Autodesk Inventor part; units mm, degrees
ref_plane "YZ Plane" through (0, 0, 0) normal (1, 0, 0) x (0, 1, 0)
ref_plane "XZ Plane" through (0, 0, 0) normal (0, 1, 0) x (-1, 0, 0)
ref_plane "XY Plane" through (0, 0, 0) normal (0, 0, 1) x (1, 0, 0)
sketch "Sketch1" plane through (0, 0, 0) normal (0, 0, 1) x (1, 0, 0)
  line L0 (-25.4, 25.4) -> (25.4, 25.4)
  line L1 (25.4, 25.4) -> (25.4, -25.4)
  line L2 (25.4, -25.4) -> (-25.4, -25.4)
  line L3 (-25.4, -25.4) -> (-25.4, 25.4)
  line L4 (24.638, 24.638) -> (-24.638, 24.638)
  line L5 (-24.638, 24.638) -> (-24.638, -24.638)
  line L6 (-24.638, -24.638) -> (24.638, -24.638)
  line L7 (24.638, -24.638) -> (24.638, 24.638)
  point P0 (0, 0)
  point P1 (0, 25.4)
  point P2 (25.4, 0)
  dimension "d0" = 50.8
  dimension "d1" = 50.8
  dimension "d2" = 0.762
extrude "Extrusion1" add sketch "Sketch1" along normal blind 279.4
sketch "Sketch2" plane through (25.4, -25.4, 0) normal (1, 0, 0) x (0, 0, -1)
  line L0 (0, 50.8) -> (-279.4, 50.8)
  line L1 (-279.4, 0) -> (-228.6, 0)
  line L2 (-228.6, 0) -> (-228.6, 50.8)
  line L3 (-228.6, 50.8) -> (-279.4, 50.8)
  line L4 (-279.4, 50.8) -> (-279.4, 0)
  line L5 (-278.638, 0.762) -> (-229.362, 0.762)
  line L6 (-229.362, 0.762) -> (-229.362, 50.038)
  line L7 (-229.362, 50.038) -> (-278.638, 50.038)
  line L8 (-278.638, 50.038) -> (-278.638, 0.762)
  point P0 (0, 25.4)
  dimension "d5" = 50.8
  dimension "d6" = 0.762
extrude "Extrusion2" add sketch "Sketch2" along normal blind 88.9
sketch "Sketch3" plane through (0, 0, 279.4) normal (0, 0, 1) x (1, 0, 0)
  point P0 (0, 0)
sketch "Sketch4" plane through (0, 0, 279.4) normal (0, 0, 1) x (1, 0, 0)
  line L0 (-25.4, -25.4) -> (114.3, -25.4)
  line L1 (114.3, 25.4) -> (63.5, 25.4)
  line L2 (63.5, 25.4) -> (63.5, -25.4)
  line L3 (63.5, -25.4) -> (114.3, -25.4)
  line L4 (114.3, -25.4) -> (114.3, 25.4)
  line L5 (113.538, 24.638) -> (64.262, 24.638)
  line L6 (64.262, 24.638) -> (64.262, -24.638)
  line L7 (64.262, -24.638) -> (113.538, -24.638)
  line L8 (113.538, -24.638) -> (113.538, 24.638)
  point P0 (0, 0)
  dimension "d9" = 50.8
  dimension "d10" = 0.762
extrude "Extrusion3" add sketch "Sketch4" along normal blind 177.8
properties part number "Side Rail"
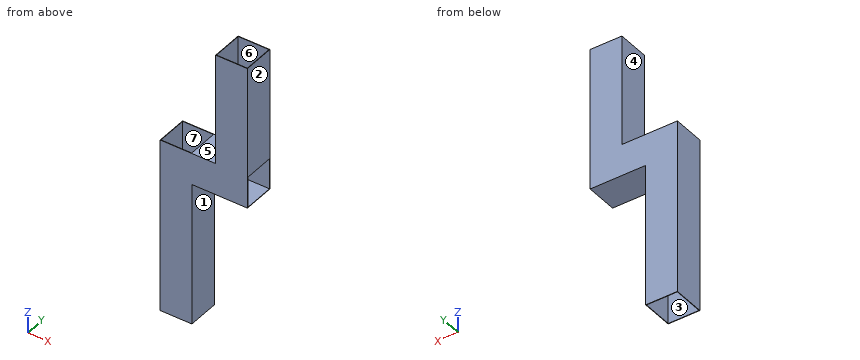
Input: part model. Units: mm. Frame: model coordinates. Face numbers are marked on the shaded views. A direction names the side the tool comes from. Round coordinates to 2 decimals unless told otherwise and drop trailing zeros. Order: outer loops, then holes, each group sorted by start corner. A loop starts at its lowest first (then second) coordinate and runs counter-clockwise, first axis right, second up. Notation, with made-up numbers: (54.25, -4) - (70.25, -4) arc R18 ccw to (70.25, 13) - close; hole circle Ø3 at (-15.75, 9). An arc over 180 degrees is marked (long way). One line per question, with ' | ' between items. Start each with the question number.
1) Ray query, probe 1 along Y at (x, z) = (95, 422.5); probe 2 along Z at (x, y) = (47, -5). Return the intervals inside material, ascending.
2) Cut plane D-D, the plane x = 9. Return the cut outline in (y, z), then the cut area to 3 significant figures.
3) Pull-direction query (X, two-part tool) for the marked faces 4, 5, 6 and 7; classes: +X half, -X half, draft (parallel to the pull), parting line (faces both ways), or undercut.
4) Set-up query: the marked faces 1, 2 and 3. Return all of +Z, -Z, +X, -X, +Y, -Y with unobstructed straight access to the full face (end or side cutting, diameter ignored); none if empty.
5) Cut plane C-C, the plane z = 425.5. Return the cut outline in (x, y), then the cut area to 3 significant figures.
6) Cut plane B-B, the plane x = 71. Return the cut outline in (y, z).
7) Contact query for flat-ended pins moving along their axis: P1, Ø15, axis at y = 6.5, z = 126, coming from the +X side; P2, Ø5, axis at x = 23.5, y = 11, coming from the +Z side; P3, Ø12, axis at x = 61, y = -7, coming from the -Z side. Output: stop coordinate, or through.
8) Cut plane A-A, the plane y = 16. Return the cut outline in (x, z), then the cut area to 3 significant figures.
Worked out:
1) probe 1: y = -25.4 to -24.64, 24.64 to 25.4 | probe 2: z = 228.6 to 229.36, 278.64 to 279.4
2) outline: (-25.4, 0) - (-24.64, 0) - (-24.64, 279.4) - (-25.4, 279.4) - close; (24.64, 0) - (25.4, 0) - (25.4, 279.4) - (24.64, 279.4) - close | area: 426 mm^2
3) face 4: -X half | face 5: draft | face 6: undercut | face 7: undercut
4) face 1: -Z, +X, +Y, -Y | face 2: +Z, -Z, +X, +Y, -Y | face 3: +Z, -Z
5) outline: (63.5, -25.4) - (114.3, -25.4) - (114.3, 25.4) - (63.5, 25.4) - close; hole (64.26, -24.64) - (113.54, -24.64) - (113.54, 24.64) - (64.26, 24.64) - close | area: 153 mm^2
6) outline: (-25.4, 228.6) - (25.4, 228.6) - (25.4, 457.2) - (24.64, 457.2) - (24.64, 279.4) - (-24.64, 279.4) - (-24.64, 457.2) - (-25.4, 457.2) - close; hole (-24.64, 229.36) - (24.64, 229.36) - (24.64, 278.64) - (-24.64, 278.64) - close
7) P1: stops at x = 25.4 | P2: stops at z = 279.4 | P3: stops at z = 228.6
8) outline: (-25.4, 0) - (-24.64, 0) - (-24.64, 279.4) - (-25.4, 279.4) - close; (24.64, 0) - (25.4, 0) - (25.4, 228.6) - (114.3, 228.6) - (114.3, 229.36) - (25.4, 229.36) - (25.4, 278.64) - (114.3, 278.64) - (114.3, 457.2) - (113.54, 457.2) - (113.54, 279.4) - (64.26, 279.4) - (64.26, 457.2) - (63.5, 457.2) - (63.5, 279.4) - (24.64, 279.4) - close | area: 832 mm^2
